Check sheet for the modelled part. Datum: model origin and axes. Units: mm. Face numbers are marked on the shaded views. A direction names the side the tool comes from. Round coordinates to 2 decimals unless told otherwise and drop trailing zeros. Write each loop counter-clockwise with the first axis right and the second up, starting at its lowest first coordinate (ties: lowest second). Pieces come first, ordered by that corner, then holes.
Item 1: Cross-section at A-A on z = 1.25. Enter the section's corners in (x, y), plus the area to 3 significant figures.
Item 2: Material ranges on line 1 (X direction, y = -0.75, z = 6); line 2 (X direction, y = 1.5, z = 3.25); line 3 (Z direction, x = -9, y = 0), recorded low to high.
Item 3: Go/stop test with flat-tipped pins: pin 1 Ø3.5 at (x, y) = (-56, -0.5) entering from +Z; pin 2 Ø2 at (x, z) = (29, 5) entering from +Y; pin 3 Ø1.6 at (y, z) = (-2, 6) entering from -X. Record where each tip stops, or that it passes through.
Item 4: Cross-section at B-B on y = -2. Enter the section's corners in (x, z), plus the area to 3 significant figures.
Item 5: Cross-section at C-C on x = -30. Enter the section's corners in (y, z), plus the area to 3 significant figures.
Item 6: Tool access check on the marked faces 1, 2 and 3. Record the directions out of +Z, -Z, +X, -X, +Y, -Y that give a thin tool (end or side, any length) a straight path to the whole face; none if there is none.
from build123d import *

# Parameters (mm, degrees)
BOSS_EXTRU_1_DEPTH = 5
ESQUISSE3_W        = 13
ESQUISSE3_H        = 5
ESQUISSE3_H_2      = 4
BOSS_EXTRU_2_DEPTH = 2


with BuildPart() as part:
    # Base pièce → Boss.-Extru.1 (new body)
    with BuildSketch(Plane.XY):
        with BuildLine():
            Line((0, 0), (15, 0))
            Line((15, 0), (15, 1))
            Line((15, 1), (68, 1))
            Line((68, 1), (68, -4))
            Line((68, -4), (-54, -4))
            ThreePointArc((-54, -4), (-55.464466094, -0.464466094), (-59, 1))
            Line((-59, 1), (-59, 3))
            Line((-59, 3), (-52, 3))
            Line((-52, 3), (-52, 1))
            Line((-52, 1), (0, 1))
            Line((0, 1), (0, 0))
        make_face()
    extrude(amount=BOSS_EXTRU_1_DEPTH)

    # Esquisse3 → Boss.-Extru.2 (add)
    with BuildSketch(Plane.XY.offset(5)):
        with Locations((-43.5, -1.5)):
            Rectangle(ESQUISSE3_W, ESQUISSE3_H)
        with Locations((7.5, -2)):
            Rectangle(ESQUISSE3_W, ESQUISSE3_H_2)
        with Locations((60.5, -1.5)):
            Rectangle(ESQUISSE3_W, ESQUISSE3_H)
    extrude(amount=BOSS_EXTRU_2_DEPTH)


solid = part.part
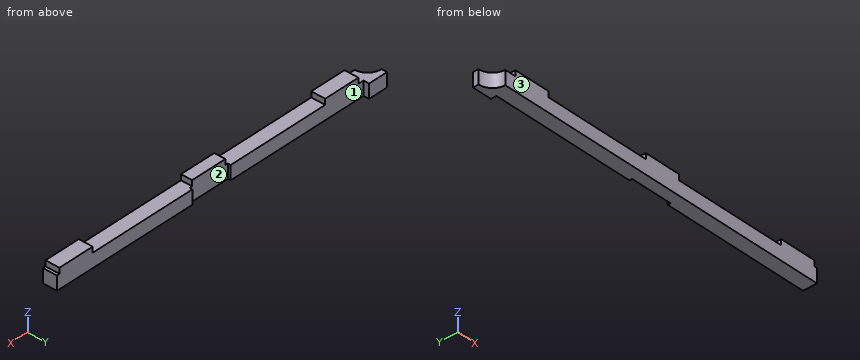
Response values:
1. outline: (-59, 1) arc R5 cw to (-54, -4) - (68, -4) - (68, 1) - (15, 1) - (15, 0) - (0, 0) - (0, 1) - (-52, 1) - (-52, 3) - (-59, 3) - close
1. area: 614 mm2
2. line 1: x = -50 to -37, 1 to 14, 54 to 67
2. line 2: x = -59 to -52
2. line 3: z = 0 to 5
3. pin 1: stops at z = 5
3. pin 2: stops at y = 1
3. pin 3: stops at x = -50
4. outline: (-54.42, 0) - (68, 0) - (68, 5) - (67, 5) - (67, 7) - (54, 7) - (54, 5) - (14, 5) - (14, 7) - (1, 7) - (1, 5) - (-37, 5) - (-37, 7) - (-50, 7) - (-50, 5) - (-54.42, 5) - close
4. area: 690 mm2
5. outline: (-4, 0) - (1, 0) - (1, 5) - (-4, 5) - close
5. area: 25.0 mm2
6. face 1: +Z, -Z, +X, +Y
6. face 2: +Z, -Z, +Y
6. face 3: +Z, -Z, +X, -X, -Y
